Autodesk Inventor part; units mm, degrees
ref_plane "YZ Plane" through (0, 0, 0) normal (1, 0, 0) x (0, 1, 0)
ref_plane "XZ Plane" through (0, 0, 0) normal (0, 1, 0) x (-1, 0, 0)
ref_plane "XY Plane" through (0, 0, 0) normal (0, 0, 1) x (1, 0, 0)
sketch "スケッチ1" plane through (0, 0, 0) normal (0, 0, 1) x (1, 0, 0)
  line L0 (0, 0) -> (132.465, 0) construction
  line L1 (0, -5) -> (132.465, -5)
  line L2 (132.465, 5) -> (0, 5)
  arc A0 (0, 5) -> (0, -5) centre (0, 0) ccw
  arc A1 (132.465, -5) -> (132.465, 5) centre (132.465, 0) ccw
  circle A2 centre (132.465, 0) radius 4.5
  circle A3 centre (0, 0) radius 5
  line L3 (0.0189, 5) -> (132.482, 4.5)
  line L4 (132.482, -4.5) -> (0.0189, -5)
  point P0 (66.2325, 0)
  point P1 (15, 0)
  point P2 (30, 0)
  point P3 (72.465, 0)
  point P4 (87.465, 0)
  point P5 (102.465, 0)
  point P6 (117.465, 0)
  point P7 (45, 0)
  point P8 (60, 0)
  dimension "d0" = 132.465
  dimension "d1" = 10
  dimension "d2" = 9
  dimension "d3" = 10
  dimension "d4" = 15
  dimension "d5" = 15
  dimension "d6" = 15
  dimension "d7" = 15
  dimension "d8" = 15
  dimension "d9" = 15
  dimension "d10" = 15
  dimension "d11" = 15
extrude "押し出し1" add sketch "スケッチ1" against normal blind 5 contours A0 L2 A3 L1 | A3 L3 A2 L4 | A2
hole "穴1" at (15, 0, 0) at (30, 0, 0) at (72.465, 0, 0) at (87.465, 0, 0) at (102.465, 0, 0) at (117.465, 0, 0) at (45, 0, 0) at (60, 0, 0) at (132.465, 0, 0) at (0, 0, 0) direction (0, 0, -1) diameter 3 depth 12 tip angle 118
sketch "スケッチ2" plane through (0, 0, 0) normal (0, 0, 1) x (1, 0, 0)
  circle A0 centre (132.465, 0) radius 1.5
  circle A1 centre (45, 0) radius 1.5
  circle A2 centre (102.465, 0) radius 1.5
  circle A3 centre (72.465, 0) radius 1.5
  circle A4 centre (15, 0) radius 1.5
  circle A5 centre (30, 0) radius 1.5
  circle A6 centre (87.465, 0) radius 1.5
  circle A7 centre (117.465, 0) radius 1.5
  circle A8 centre (60, 0) radius 1.5
  circle A9 centre (0, 0) radius 1.5
  line L0 (132.482, -4.5) -> (0.0189, -5)
  arc A10 (0.0189, 5) -> (0.0189, -5) centre (0, 0) ccw
  line L1 (0.0189, 5) -> (132.482, 4.5)
  arc A11 (132.482, -4.5) -> (132.482, 4.5) centre (132.465, 0) ccw
sketch "スケッチ3" plane through (0, 0, 0) normal (0, 0, 1) x (1, 0, 0)
  circle A0 centre (132.465, 0) radius 1.5
  circle A1 centre (45, 0) radius 1.5
  circle A2 centre (102.465, 0) radius 1.5
  circle A3 centre (72.465, 0) radius 1.5
  circle A4 centre (15, 0) radius 1.5
  circle A5 centre (30, 0) radius 1.5
  circle A6 centre (87.465, 0) radius 1.5
  circle A7 centre (117.465, 0) radius 1.5
  circle A8 centre (60, 0) radius 1.5
  circle A9 centre (0, 0) radius 1.5
  line L0 (132.482, -4.5) -> (0.0189, -5)
  arc A10 (0.0189, 5) -> (0.0189, -5) centre (0, 0) ccw
  line L1 (0.0189, 5) -> (132.482, 4.5)
  arc A11 (132.482, -4.5) -> (132.482, 4.5) centre (132.465, 0) ccw
  line L2 (132.4707, 1.5) -> (0.0075, 2)
  arc A12 (0.0075, 2) -> (0.0075, -2) centre (0, 0) ccw
  line L3 (0.0075, -2) -> (132.4707, -1.5)
  arc A13 (132.4707, -1.5) -> (132.4707, 1.5) centre (132.465, 0) ccw
  circle A14 centre (0, 0) radius 4.5
  circle A15 centre (15, 0) radius 4.5
  circle A16 centre (30, 0) radius 4.5
  circle A17 centre (45, 0) radius 4.5
  circle A18 centre (60, 0) radius 4.5
  circle A19 centre (72.465, 0) radius 4.5
  circle A20 centre (87.465, 0) radius 4.5
  circle A21 centre (102.465, 0) radius 4.5
  circle A22 centre (117.465, 0) radius 4.5
  circle A23 centre (132.465, 0) radius 4.5
  point P0 (98.2702, -1.6291)
  point P1 (98.2702, 1.6291)
  point P2 (91.65, 1.6541)
  point P3 (91.65, -1.6541)
  point P4 (113.2487, -1.5725)
  point P5 (113.2487, 1.5725)
  point P6 (106.6719, 1.5974)
  point P7 (106.6719, -1.5974)
  point P8 (128.2281, -1.516)
  point P9 (128.2281, 1.516)
  point P10 (121.693, 1.5407)
  point P11 (121.693, -1.5407)
  point P12 (83.2926, -1.6856)
  point P13 (83.2926, 1.6856)
  point P14 (76.6271, 1.7108)
  point P15 (76.6271, -1.7108)
  point P16 (68.3159, -1.7421)
  point P17 (68.3159, 1.7421)
  point P18 (64.1424, 1.7579)
  point P19 (64.1424, -1.7579)
  point P20 (55.871, -1.7891)
  point P21 (55.871, 1.7891)
  point P22 (49.1179, 1.8146)
  point P23 (49.1179, -1.8146)
  point P24 (40.8959, -1.8456)
  point P25 (40.8959, 1.8456)
  point P26 (34.0924, 1.8713)
  point P27 (34.0924, -1.8713)
  point P28 (25.9218, -1.9022)
  point P29 (25.9218, 1.9022)
  point P30 (19.066, 1.928)
  point P31 (19.066, -1.928)
  point P32 (10.9486, -1.9587)
  point P33 (10.9486, 1.9587)
  point P34 (4.0386, 1.9848)
  point P35 (4.0386, -1.9848)
  dimension "d21" = 3
  dimension "d22" = 3
  dimension "d23" = 3
  dimension "d24" = 3
  dimension "d25" = 3
  dimension "d26" = 3
  dimension "d27" = 3
  dimension "d28" = 3
  dimension "d29" = 3
  dimension "d30" = 3
  dimension "d31" = 3
extrude "押し出し2" cut sketch "スケッチ3" against normal blind 4 contours A23 L3 A22 L2 | A22 L3 A21 L2 | A21 L3 A20 L2 | A20 L3 A19 L2 | A19 L3 A18 L2 | A18 L3 A17 L2 | A17 L3 A16 L2 | A16 L3 A15 L2 | A15 L3 A14 L2
fillet "フィレット1" radius 1 36 edges at (4.0386, -1.9848, -2) (4.0386, 1.9848, -2) (10.9486, 1.9587, -2) (10.9486, -1.9587, -2) (19.066, -1.928, -2) (19.066, 1.928, -2) (25.9218, 1.9022, -2) (25.9218, -1.9022, -2) (40.8959, 1.8456, -2) (40.8959, -1.8456, -2) (34.0924, 1.8713, -2) (34.0924, -1.8713, -2) (55.871, 1.7891, -2) (55.871, -1.7891, -2) (49.1179, 1.8146, -2) (49.1179, -1.8146, -2) (68.3159, 1.7421, -2) (68.3159, -1.7421, -2) (64.1424, 1.7579, -2) (64.1424, -1.7579, -2) (83.2926, 1.6856, -2) (83.2926, -1.6856, -2) (76.6271, 1.7108, -2) (76.6271, -1.7108, -2) (98.2702, 1.6291, -2) (98.2702, -1.6291, -2) (91.65, 1.6541, -2) (91.65, -1.6541, -2) (113.2487, 1.5725, -2) (113.2487, -1.5725, -2) (106.6719, 1.5974, -2) (106.6719, -1.5974, -2) (128.2281, 1.516, -2) (128.2281, -1.516, -2) (121.693, 1.5407, -2) (121.693, -1.5407, -2)
properties part number "カウンター 中間部" material "アルミニウム 7075"
Can you work these out from the model? Positions are in its coordinate system, mm. A direction names the side the tool comes from. Coordinates: 2 decimals unless noted, no trailing zeros. Loops run counter-clockwise (first coordinate to the right, second up) from the corner with the lowest first, then second, coordinate; pieces in that order, holes last. Notation, with made-up numbers: M 11,49 L 24,49 A30 ccw 24,88 Z; hole C -27,10.5 d9. An arc over 180 degrees is marked long. Put each result on its own line as item: value. Start each with the question number.
(1) Imagine slicing it at B-B on x = 60. List the corners of the cut face in (y, z) for me, and give its area (3 significant figures).
(2) Imagine slicing it at A-A on x = 15. List the corners of the cut face in (y, z) for me, and give its area (3 significant figures).
(3) Will these pins go through, and if not, where does the flat tip stop? pin 1 Ø1.8 at (x, y) = (0, 0) entering from +Z; pin 2 Ø1.2 at (x, y) = (23, 0) entering from +Z; pin 3 Ø1 at (x, z) = (107.5, -1.5) entering from +Y; pin 4 Ø2 at (y, z) = (3.5, -2) entering from -X.
(4) We'd pull the mould along Y, two halves only. Please class faces 1 (the face through (131.2, -0.806, -2.535)), 2 (the face through (65, 0, -5)), 3 (the face through (-5, 0, -2)): +Y half, -Y half, draft (parallel to the pull), parting line (faces both ways), or undercut.
(5) Imagine slicing it at C-C on z = -2.55. Give the number of separate pieces and of enclosed holes in the cut face, and give its area (3 significant figures).
(6) I need wall thicknesses on probe 1 along Z at (x, y) = (8, 1); probe 2 along Y at (x, z) = (88, -3.2); probe 3 along Y at (x, z) = (30, -3.1). Which ranges of each line are inside material? Lowest first, please.
(7) Which directions (+Z, -Z, +X, -X, +Y, -Y) give clear straight access to the entire face, cutting with the end or side of a thin tool? Please do faces 4 (the face through (46.464, 0.325, -2.535)), 5 (the face through (37, 0, -4)).
Worked answers:
1. outline: M -4.77,-5 L -1.5,-5 L -1.5,0 L -4.77,0 Z; M 1.5,-5 L 4.77,-5 L 4.77,0 L 1.5,0 Z
1. area: 32.7 mm2
2. outline: M -4.94,-5 L -1.5,-5 L -1.5,0 L -4.94,0 Z; M 1.5,-5 L 4.94,-5 L 4.94,0 L 1.5,0 Z
2. area: 34.4 mm2
3. pin 1: passes through
3. pin 2: stops at z = -4
3. pin 3: stops at y = 4.6
3. pin 4: stops at x = -4.33
4. face 1: undercut
4. face 2: draft
4. face 3: parting line
5. separate pieces: 1
5. enclosed holes: 19
5. area: 1,080 mm2
6. probe 1: z = -5 to -4
6. probe 2: y = -4.67 to -1.4, 1.4 to 4.67
6. probe 3: y = -4.89 to -1.5, 1.5 to 4.89
7. face 4: +Z, -Z
7. face 5: +Z
